The model under review builds one solid part; all positions refer to its coordinate system, in mm. Give positions to 0.01 mm unless a question says otherwise; leave off trailing zeros. Order: outer loops, then holes, each group sorted by start corner. A loop starts at its lowest first (then second) coordinate and runs counter-clockwise, first axis right, second up.
```python
from build123d import *

# Parameters (mm, degrees)
SKETCH1_W           = 105
SKETCH1_H           = 100
BOSS_EXTRUDE1_DEPTH = 2.5
SKETCH3_W           = 4
SKETCH3_H           = 4
BOSS_EXTRUDE2_DEPTH = 4
SKETCH5_W           = 85
SKETCH5_H           = 80
CUT_EXTRUDE2_DEPTH  = 4
SKETCH6_R           = 15
BOSS_EXTRUDE3_DEPTH = 2.5
SKETCH7_W           = 5
SKETCH7_H           = 5
CUT_EXTRUDE3_DEPTH  = 2.5
BOSS_EXTRUDE4_DEPTH = 2.5
EXTRUDE_THIN2_DEPTH = 2.5
SKETCH10_R          = 3
CUT_EXTRUDE5_DEPTH  = 2.5
SKETCH11_W          = 3
SKETCH11_H          = 3
CUT_EXTRUDE6_DEPTH  = 2.5
SKETCH12_R          = 10
CUT_EXTRUDE7_DEPTH  = 10


with BuildPart() as part:
    # Sketch1 → Boss-Extrude1 (new body)
    with BuildSketch(Plane(origin=(0, 0, 0), x_dir=(1, 0, 0), z_dir=(0, 1, 0))):
        Rectangle(SKETCH1_W, SKETCH1_H)
    extrude(amount=BOSS_EXTRUDE1_DEPTH)

    # Sketch3 → Boss-Extrude2 (add)
    with BuildSketch(Plane(origin=(0, 2.5, 0), x_dir=(1, 0, 0), z_dir=(0, 1, 0))):
        with Locations((-50.5, 48)):
            Rectangle(SKETCH3_W, SKETCH3_H)
        with Locations((50.5, 48)):
            Rectangle(SKETCH3_W, SKETCH3_H)
        with Locations((50.5, -48)):
            Rectangle(SKETCH3_W, SKETCH3_H)
        with Locations((-50.5, -48)):
            Rectangle(SKETCH3_W, SKETCH3_H)
    extrude(amount=BOSS_EXTRUDE2_DEPTH)

    # Sketch5 → Cut-Extrude2 (cut)
    with BuildSketch(Plane(origin=(0, 2.5, 0), x_dir=(1, 0, 0), z_dir=(0, 1, 0))):
        Rectangle(SKETCH5_W, SKETCH5_H)
    extrude(amount=-CUT_EXTRUDE2_DEPTH, mode=Mode.SUBTRACT)

    # Sketch8 → Boss-Extrude4 (add)
    with BuildSketch(Plane(origin=(0, 2.5, 0), x_dir=(1, 0, 0), z_dir=(0, 1, 0))):
        with BuildLine():
            Line((-42.5, -40), (-27.220069463, -40))
            ThreePointArc((-27.220069463, -40), (-31.695457502, -29.195457502), (-42.5, -24.720069463))
            Line((-42.5, -24.720069463), (-42.5, -40))
        make_face()
        with BuildLine():
            ThreePointArc((-42.5, 24.720069463), (-31.695457502, 29.195457502), (-27.220069463, 40))
            Line((-27.220069463, 40), (-42.5, 40))
            Line((-42.5, 40), (-42.5, 24.720069463))
        make_face()
        with BuildLine():
            Line((42.5, 40), (27.220069463, 40))
            ThreePointArc((27.220069463, 40), (31.695457502, 29.195457502), (42.5, 24.720069463))
            Line((42.5, 24.720069463), (42.5, 40))
        make_face()
        with BuildLine():
            ThreePointArc((42.5, -24.720069463), (31.695457502, -29.195457502), (27.220069463, -40))
            Line((27.220069463, -40), (42.5, -40))
            Line((42.5, -40), (42.5, -24.720069463))
        make_face()
    extrude(amount=-BOSS_EXTRUDE4_DEPTH)



with BuildPart() as body_2:
    # Sketch6 → Boss-Extrude3 (new body)
    with BuildSketch(Plane(origin=(0, 2.5, 0), x_dir=(1, 0, 0), z_dir=(0, 1, 0))):
        with Locations(Location((0, 0, 0), (0, 0, 270))):
            Circle(SKETCH6_R)
    extrude(amount=-BOSS_EXTRUDE3_DEPTH)

    # Sketch7 → Cut-Extrude3 (cut)
    with BuildSketch(Plane(origin=(0, 2.5, 0), x_dir=(1, 0, 0), z_dir=(0, 1, 0))):
        Rectangle(SKETCH7_W, SKETCH7_H)
    extrude(amount=-CUT_EXTRUDE3_DEPTH, mode=Mode.SUBTRACT)


with BuildPart() as part_1:
    add(part.part)

    add(body_2.part)  # Extrude-Thin2 merges body 2
    # Sketch9 → Extrude-Thin2 (add)
    with BuildSketch(Plane(origin=(0, 2.5, 0), x_dir=(1, 0, 0), z_dir=(0, 1, 0))):
        Polygon((-1.035533906, -6.035533906), (34.46870341, -41.539771222), (41.539771222, -34.46870341), (6.035533906, 1.035533906), align=None)
        Polygon((-11.285533906, -4.214466094), (-41.539771222, -34.46870341), (-34.46870341, -41.539771222), (-4.214466094, -11.285533906), align=None)
        Polygon((11.285533906, 4.214466094), (41.539771222, 34.46870341), (34.46870341, 41.539771222), (4.214466094, 11.285533906), align=None)
        Polygon((-4.214466094, 11.285533906), (-34.46870341, 41.539771222), (-41.539771222, 34.46870341), (-11.285533906, 4.214466094), align=None)
    extrude(amount=-EXTRUDE_THIN2_DEPTH)

    # Sketch10 → Cut-Extrude5 (cut)
    with BuildSketch(Plane(origin=(0, 2.5, 0), x_dir=(1, 0, 0), z_dir=(0, 1, 0))):
        with Locations(Location((38.5, 36, 0), (0, 0, 270))):
            Circle(SKETCH10_R)
        with Locations(Location((-38.5, 36, 0), (0, 0, 90))):
            Circle(SKETCH10_R)
        with Locations(Location((38.5, -36, 0), (0, 0, 90))):
            Circle(SKETCH10_R)
        with Locations(Location((-38.5, -36, 0), (0, 0, 270))):
            Circle(SKETCH10_R)
    extrude(amount=-CUT_EXTRUDE5_DEPTH, mode=Mode.SUBTRACT)

    # Sketch11 → Cut-Extrude6 (cut)
    with BuildSketch(Plane(origin=(0, 2.5, 0), x_dir=(1, 0, 0), z_dir=(0, 1, 0))):
        with Locations((40.657260224, -44.752137111)):
            Rectangle(SKETCH11_W, SKETCH11_H)
        with Locations((35.291405318, -44.752137111)):
            Rectangle(SKETCH11_W, SKETCH11_H)
    extrude(amount=-CUT_EXTRUDE6_DEPTH, mode=Mode.SUBTRACT)

    # Sketch12 → Cut-Extrude7 (cut)
    with BuildSketch(Plane(origin=(0, 2.5, 0), x_dir=(1, 0, 0), z_dir=(0, 1, 0))):
        with Locations(Location((0, 0, 0), (0, 0, 270))):
            Circle(SKETCH12_R)
    extrude(amount=-CUT_EXTRUDE7_DEPTH, mode=Mode.SUBTRACT)


solid = part_1.part
```
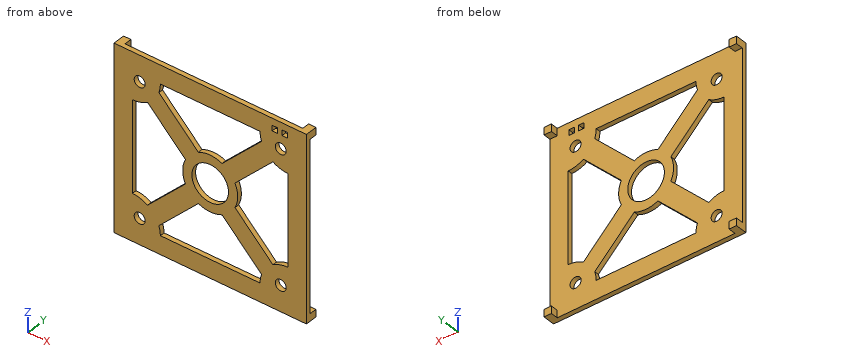
Item 1: Clearance check with flat-ended pins moving along their axes: pin 1 Ø3.5 at (x, z) = (-38.5, 36) entering from -Y; pin 2 Ø12 at (x, z) = (8, -4.5) entering from +Y. State where each tip first meets the part, or that it passes through.
Values found:
pin 1: passes through
pin 2: stops at y = 2.5
Item 2: For line 1 (X direction, y = 1.5, z = 45); line 2 (Z direction, x = 34, y = 2.25); line 3 (X direction, y = 1.75, z = -36), list the stretches that pass through material, from the lowest coordinate up.
Values found:
line 1: x = -52.5 to 33.79, 36.79 to 39.16, 42.16 to 52.5
line 2: z = -50 to -26.93, 26.93 to 43.25, 46.25 to 50
line 3: x = -52.5 to -41.5, -35.5 to -27.75, 27.75 to 35.5, 41.5 to 52.5
Item 3: Take a section at D-D (x = -31.5). Give the boundary of the cut face in (y, z), and give its area (3 significant figures).
Values found:
outline: (0, -50) - (2.5, -50) - (2.5, -24.43) - (0, -24.43) - close; (0, 24.43) - (2.5, 24.43) - (2.5, 50) - (0, 50) - close
area: 128 mm2
Item 4: Take a section at A-A (x = 0). Give the boundary of the cut face in (y, z), and give its area (3 significant figures).
Values found:
outline: (0, -50) - (2.5, -50) - (2.5, -40) - (0, -40) - close; (0, -15) - (2.5, -15) - (2.5, -10) - (0, -10) - close; (0, 10) - (2.5, 10) - (2.5, 15) - (0, 15) - close; (0, 40) - (2.5, 40) - (2.5, 50) - (0, 50) - close
area: 75.0 mm2
Item 5: Take a section at B-B (y = 4.25). Give the boundary of the cut face in (x, z), and give its area (3 significant figures).
Values found:
outline: (-52.5, -50) - (-48.5, -50) - (-48.5, -46) - (-52.5, -46) - close; (-52.5, 46) - (-48.5, 46) - (-48.5, 50) - (-52.5, 50) - close; (48.5, -50) - (52.5, -50) - (52.5, -46) - (48.5, -46) - close; (48.5, 46) - (52.5, 46) - (52.5, 50) - (48.5, 50) - close
area: 64.0 mm2
Item 6: Take a section at C-C (z = 28.5). Give the boundary of the cut face in (x, y), and give its area (3 significant figures).
Values found:
outline: (-52.5, 0) - (-21.43, 0) - (-21.43, 2.5) - (-52.5, 2.5) - close; (21.43, 0) - (52.5, 0) - (52.5, 2.5) - (21.43, 2.5) - close
area: 155 mm2
